```python
from build123d import *

# Parameters (mm, degrees)
VERRUNDUNG1_R = 0.8
VERRUNDUNG2_R = 0.2


with BuildPart() as part:
    # Skizze1 → Rotation1 (revolve)
    with BuildSketch(Plane(origin=(0, 0, 0), x_dir=(0, 0, -1), z_dir=(1, 0, 0)), mode=Mode.PRIVATE) as rotation1_sk:
        Polygon((0, 2.5), (0, 1), (6, 1), (6, 2), (3.5, 2), (3.5, 2.5), align=None)
    revolve(rotation1_sk.sketch.rotate(Axis((0, 0, 0), (0, 0, -1)), 90), axis=Axis((0, 0, 0), (0, 0, -1)))

    # Verrundung1
    verrundung1_edges = [part.edges().sort_by_distance(p)[0] for p in [
        (-1, 0, -6),
    ]]
    fillet(verrundung1_edges, radius=VERRUNDUNG1_R)

    # Verrundung2
    verrundung2_edges = [part.edges().sort_by_distance(p)[0] for p in [
        (-2, 0, -6),
    ]]
    fillet(verrundung2_edges, radius=VERRUNDUNG2_R - 0.0001)  # a hair under: the kernel refuses the full size


solid = part.part
```
Check sheet for the modelled part. Datum: model origin and axes. Units: mm. Round coordinates to 2 decimals unless told otherwise and drop trailing zeros. Loops run counter-clockwise (first coordinate to the right, second up) from the corner with the lowest first, then second, coordinate; pieces in that order, holes last. Notation, with made-up numbers: M 40.5,-0.5 L 75.5,-0.5 A29 ccw 75.5,22.5 Z; hole C 88.5,-38.5 d4. An arc over 180 degrees is marked long. Answer as a JSON object with one key per item and string values.
1. Section check C-C (z = -5.05). Record the boundary of the cut face in (x, y).
Reply:
{"outline": "C 0,0 d4; hole C 0,0 d2"}
2. Scan lines: line 1 (Y direction, x = 0, z = -1.3); line 2 (Z direction, x = 1.75, y = 1.45); line 3 (Y direction, x = -0.4, z = -4.3). Record each from-to range of solid material in increasing order.
Reply:
{"line 1": "y = -2.5 to -1, 1 to 2.5", "line 2": "z = -3.5 to 0", "line 3": "y = -1.96 to -0.92, 0.92 to 1.96"}
3. Gauge pin test, flat end, axial feed: P1, Ø1.5, axis at x = 1, z = -1, coming from the +Y side. Record the tip position at first contact, or that the pin passes through.
Reply:
{"P1": "stops at y = 2.49"}
4. Mould release check, pull along X, two halves, no side actions. Record for faces 1 (the cylindrical face through (0, 2, -5)), 2 (the cylindrical face through (0, 1, -3)), 3 (the flat face through (1, -2, -3.5)): pulls with the +X half, pulls with the -X half, needs draft (parallel to the pull), parting line crosses it, or undercut.
Reply:
{"face 1": "parting line crosses it", "face 2": "undercut", "face 3": "needs draft"}
5. Section check D-D (z = -1.4). Record the boundary of the cut face in (x, y), plus the area to 3 significant figures.
Reply:
{"outline": "C 0,0 d5; hole C 0,0 d2", "area": "16.5 mm²"}
